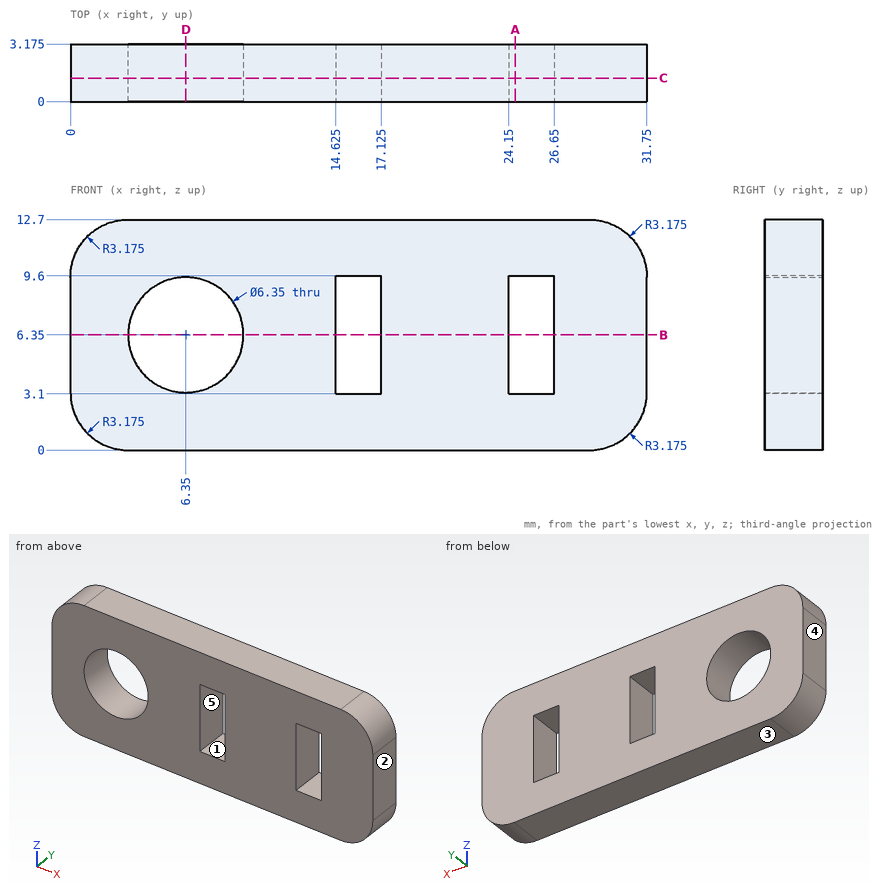
Study the drawing (mm; zero at the part's minimum x, y, z) and answer. A direction names the side the tool comes from. Give positions to 0.01 mm unless a question says otherwise; leave off trailing zeros. Write each loop counter-clockwise with the first axis right and the second up, starting at its lowest first coordinate (ties: lowest second). Pieces come first, ordered by that corner, then holes.
Item 1: Section A-A, the plane x = 24.5 is taken. Write down the section's boundary in (y, z) (3 decimals), plus the area to 3 significant figures.
Item 2: Which of the six approach directions +Z, -Z, +X, -X, +Y, -Y give full straight-line access (tool end or side, diameter ignored) to the marked faces 4 and 5?
Item 3: Determine the mould class of the marked faces 1, 2 and 3 for opening direction X: released by +X, released by -X, zero draft, split by the parting line, or undercut.
Item 4: Section C-C, the plane y = 1.3 is taken. Write down the section's boundary in (x, z) (3 decimals).
Item 5: A flat-ended cylindrical pin translates along its axis: P1, Ø1.2, axis at x = 26, y = 1.5, coming from the -Z side. Find the tip coordinate at first contact, or state that the pin passes through.
Item 6: Section B-B, the plane z = 6.35 is taken. Write down the section's boundary in (x, y) (3 decimals), plus the area to 3 significant figures.
Item 7: Find the intervals of material crossed by line 1 along Z through (x, y) = (6.35, 1.45) (3 decimals); line 2 along X through (y, z) = (2.3, 4.5) (3 decimals); line 3 along X through (y, z) = (0.45, 5.75) (3 decimals), in increasing order.
Item 8: Section D-D, the plane x = 6.35 is taken. Write down the section's boundary in (y, z) (3 decimals), plus the area to 3 significant figures.
Completed:
1. outline: (0, 0) - (3.175, 0) - (3.175, 3.1) - (0, 3.1) - close; (0, 9.6) - (3.175, 9.6) - (3.175, 12.7) - (0, 12.7) - close
1. area: 19.7 mm2
2. face 4: +Z, -Z, -X, +Y, -Y
2. face 5: +Y, -Y
3. face 1: undercut
3. face 2: released by +X
3. face 3: zero draft
4. outline: (0, 3.175) arc R3.175 ccw to (3.175, 0) - (28.575, 0) arc R3.175 ccw to (31.75, 3.175) - (31.75, 9.525) arc R3.175 ccw to (28.575, 12.7) - (3.175, 12.7) arc R3.175 ccw to (0, 9.525) - close; hole circle Ø6.35 at (6.35, 6.35); hole (14.625, 3.1) - (17.125, 3.1) - (17.125, 9.6) - (14.625, 9.6) - close; hole (24.15, 3.1) - (26.65, 3.1) - (26.65, 9.6) - (24.15, 9.6) - close
5. P1: stops at z = 0
6. outline: (0, 0) - (3.175, 0) - (3.175, 3.175) - (0, 3.175) - close; (9.525, 0) - (14.625, 0) - (14.625, 3.175) - (9.525, 3.175) - close; (17.125, 0) - (24.15, 0) - (24.15, 3.175) - (17.125, 3.175) - close; (26.65, 0) - (31.75, 0) - (31.75, 3.175) - (26.65, 3.175) - close
6. area: 64.8 mm2
7. line 1: z = 0 to 3.175, 9.525 to 12.7
7. line 2: x = 0 to 3.77, 8.93 to 14.625, 17.125 to 24.15, 26.65 to 31.75
7. line 3: x = 0 to 3.232, 9.468 to 14.625, 17.125 to 24.15, 26.65 to 31.75
8. outline: (0, 0) - (3.175, 0) - (3.175, 3.175) - (0, 3.175) - close; (0, 9.525) - (3.175, 9.525) - (3.175, 12.7) - (0, 12.7) - close
8. area: 20.2 mm2
